Build history of the part. All positions in model axes, mm. A direction names the side the tool comes from. Give positions to 0.01 mm unless a question says otherwise; leave off trailing zeros. Write each loop counter-clockwise with the first axis right and the second up, starting at its lowest first coordinate (ties: lowest second). Pieces come first, ordered by that corner, then holes.
from build123d import *

# Parameters (mm, degrees)
CROQUIS1_W              = 410
CROQUIS1_H              = 235
SALIENTE_EXTRUIR1_DEPTH = 78
CROQUIS2_W              = 377
CROQUIS2_H              = 186.930394922
CORTAR_EXTRUIR1_DEPTH   = 5
CROQUIS3_W              = 369
CROQUIS3_H              = 178.930394922
SALIENTE_EXTRUIR2_DEPTH = 8
CROQUIS5_W              = 300
CROQUIS5_H              = 99
CORTAR_EXTRUIR2_DEPTH   = 20


with BuildPart() as part:
    # Croquis1 → Saliente-Extruir1 (new body)
    with BuildSketch(Plane.XY):
        with Locations((161.576639223, 109.430394922)):
            Rectangle(CROQUIS1_W, CROQUIS1_H)
    extrude(amount=SALIENTE_EXTRUIR1_DEPTH)

    # Croquis2 → Cortar-Extruir1 (cut)
    with BuildSketch(Plane.XY.offset(78)):
        with Locations((159.076639223, 93.465197461)):
            Rectangle(CROQUIS2_W, CROQUIS2_H)
    extrude(amount=-CORTAR_EXTRUIR1_DEPTH, mode=Mode.SUBTRACT)

    # Croquis3 → Saliente-Extruir2 (add)
    with BuildSketch(Plane.XY.offset(73)):
        with Locations((159.076639223, 93.465197461)):
            Rectangle(CROQUIS3_W, CROQUIS3_H)
    extrude(amount=SALIENTE_EXTRUIR2_DEPTH)

    # Croquis5 → Cortar-Extruir2 (cut)
    with BuildSketch(Plane.XY.offset(81)):
        with Locations((156.576639223, 98.430394922)):
            Rectangle(CROQUIS5_W, CROQUIS5_H)
    extrude(amount=-CORTAR_EXTRUIR2_DEPTH, mode=Mode.SUBTRACT)


solid = part.part
(1) 3-axis set-ups, long thin cutter, end or side, ignore diameter. For faces 5 (the face through (-43.423, 108, 38)), 6 (the face through (156, 4, 77)): which of +Z, -Z, +X, -X, +Y, -Y reach the whole face in a straight line?
(2) Drop a flat-ended pin along its axis: pin 1 (6 mm diameter, centred on x = 190.5, y = 200.5, fed in from -Z). Give the stop position or say it passes through.
(3) Saw through at C-C, the plane y = 192. List the corners of the cut face in (x, z).
(4) Mould opens along Y. For faces 1 (the face through (343.577, 92, 77)), 2 (the face through (159, 111, 0)), 3 (the face through (159, 226.93, 38)), 4 (the face through (159, -8.07, 38)) say: +Y half, -Y half, draft (parallel to the pull), parting line (faces both ways), or undercut.
(5) Probe line 1 (X direction, y = 151, z = 77); line 2 (X direction, y = 89.5, z = 68); line 3 (Z direction, x = 286, y = 133). List the from-to ranges inside material, lowest first.
(6) Saw through at B-B, the plane y = 63. List the corners of the cut face in (x, z).
(7) Saw through at A-A, the plane x = 289.5. List the corners of the cut face in (y, z).
Computed values:
1. face 5: +Z, -Z, -X, +Y, -Y
1. face 6: +Z
2. pin 1: stops at z = 0
3. outline: (-43.42, 0) - (366.58, 0) - (366.58, 78) - (-43.42, 78) - close
4. face 1: undercut
4. face 2: draft
4. face 3: +Y half
4. face 4: -Y half
5. line 1: x = -43.42 to -29.42, -25.42 to 343.58, 347.58 to 366.58
5. line 2: x = -43.42 to 6.58, 306.58 to 366.58
5. line 3: z = 0 to 61
6. outline: (-43.42, 0) - (366.58, 0) - (366.58, 78) - (347.58, 78) - (347.58, 73) - (343.58, 73) - (343.58, 81) - (306.58, 81) - (306.58, 61) - (6.58, 61) - (6.58, 81) - (-25.42, 81) - (-25.42, 73) - (-29.42, 73) - (-29.42, 78) - (-43.42, 78) - close
7. outline: (-8.07, 0) - (226.93, 0) - (226.93, 78) - (186.93, 78) - (186.93, 73) - (182.93, 73) - (182.93, 81) - (147.93, 81) - (147.93, 61) - (48.93, 61) - (48.93, 81) - (4, 81) - (4, 73) - (0, 73) - (0, 78) - (-8.07, 78) - close
